```python
from build123d import *

# Parameters (mm, degrees)
F1_DEPTH  = 30.48
F2_DEPTH  = 30.48
F3_DEPTH  = 30.48
F5_DEPTH  = 661.416
F6_W      = 45.72
F6_H      = 152.3821130395
F7_DEPTH  = 222.504
F9_DEPTH  = 46.3296
F10_DEPTH = 18.288
F13_DEPTH = 296.2656
F14_DEPTH = 86.2584
F15_DEPTH = 18.288


with BuildPart() as f1:
    # F0 (on Front) → F1 (new body)
    with BuildSketch(Plane.XZ):
        Polygon((16.8911121702, 157.9167651749), (-44.0688878298, 96.9567651749), (16.8911121702, 96.9567651749), align=None)
        Polygon((16.8911121702, 96.9567651749), (-44.0688878298, 96.9567651749), (-44.0688878298, -665.0432348251), (16.8911121702, -665.0432348251), (16.8911121702, -726.0032348251), (86.011223495, -683.3165884018), (86.011223495, -646.4774608612), (43.015755713, -506.0282349586), (43.015755713, -86.7099538445), (68.1852996349, 21.7126905918), (61.4088848233, 96.9567651749), (16.8911121702, 157.9167651749), align=None)
        Polygon((16.8911121702, -665.0432348251), (-44.0688878298, -665.0432348251), (16.8911121702, -726.0032348251), align=None)
    extrude(amount=F1_DEPTH)

    # F2 (add): a face of the model
    f2_faces = [f1.faces().sort_by_distance(p)[0] for p in [
        (6.2050010019, -30.48, -294.9143233184),
    ]]
    extrude(f2_faces, amount=F2_DEPTH)

    # F3 (add): a face of the model
    f3_faces = [f1.faces().sort_by_distance(p)[0] for p in [
        (6.2050010019, -60.96, -294.9143233184),
    ]]
    extrude(f3_faces, amount=F3_DEPTH)

    # F4 (on face) → F5 (cut)
    with BuildSketch(Plane(origin=(0, 0, 0), x_dir=(-1, 0, 0), z_dir=(0, 1, 0))):
        with BuildLine():
            Line((44.0688878298, -581.2422633171), (44.0688878298, -34.1473101496))
            ThreePointArc((44.0688878298, -34.1473101496), (7.0024431669, -307.6947867334), (44.0688878298, -581.2422633171))
        make_face()
    extrude(amount=-F5_DEPTH, mode=Mode.SUBTRACT)

    # F6 (on face) → F7 (cut)
    with BuildSketch(Plane.YZ.offset(43.015755713)):
        with Locations((-68.58, -198.6809484661)):
            Rectangle(F6_W, F6_H)
    extrude(amount=-F7_DEPTH, mode=Mode.SUBTRACT)

    # F8 (on face) → F9 (cut)
    with BuildSketch(Plane(origin=(0, 0, 0), x_dir=(-1, 0, 0), z_dir=(0, 1, 0))):
        with BuildLine():
            Line((-68.1852996349, 21.7126905918), (-43.015755713, -86.7099538445))
            Line((-43.015755713, -86.7099538445), (31.0375482418, -86.7099538445))
            ThreePointArc((31.0375482418, -86.7099538445), (37.2070107283, -60.3428002224), (44.0688878298, -34.1473101496))
            Line((44.0688878298, -34.1473101496), (44.0688878298, 96.9567651749))
            Line((44.0688878298, 96.9567651749), (-16.8911121702, 157.9167651749))
            Line((-16.8911121702, 157.9167651749), (-61.4088848233, 96.9567651749))
            Line((-61.4088848233, 96.9567651749), (-68.1852996349, 21.7126905918))
        make_face()
    extrude(amount=-F9_DEPTH, mode=Mode.SUBTRACT)

    # F10 (cut): a face of the model
    f10_faces = [f1.faces().sort_by_distance(p)[0] for p in [
        (15.3196752296, 0, -444.822898096),
    ]]
    extrude(f10_faces, amount=-F10_DEPTH, mode=Mode.SUBTRACT)

    # F12 (on face) → F13 (cut)
    with BuildSketch(Plane.XZ.offset(91.44)):
        with BuildLine():
            Line((43.015755713, -390.4501199722), (43.015755713, -293.7003970146))
            ThreePointArc((43.015755713, -293.7003970146), (27.028136051, -299.6814009845), (26.5955161303, -316.7456686497))
            ThreePointArc((26.5955161303, -316.7456686497), (35.3432447647, -353.478123173), (43.015755713, -390.4501199722))
        make_face()
    extrude(amount=-F13_DEPTH, mode=Mode.SUBTRACT)

    # F11 (on face) → F14 (cut)
    with BuildSketch(Plane.YZ.offset(43.015755713)):
        with BuildLine():
            Line((-71.4861452579, -398.3681499958), (-71.4861452579, -306.9769144058))
            ThreePointArc((-71.4861452579, -306.9769144058), (-76.814746868, -292.4826164705), (-91.44, -287.5247299671))
            Line((-91.44, -287.5247299671), (-91.44, -506.0282349586))
            Line((-91.44, -506.0282349586), (-71.4861452579, -506.0282349586))
            Line((-71.4861452579, -506.0282349586), (-71.4861452579, -398.3681499958))
        make_face()
        with BuildLine():
            ThreePointArc((-27.6783167816, -287.4728058939), (-23.0664051614, -286.1317966662), (-18.288, -285.6471538544))
            Line((-18.288, -285.6471538544), (-18.288, -270.6759691181))
            ThreePointArc((-18.288, -270.6759691181), (-22.0060984175, -279.6206155123), (-27.6783167816, -287.4728058939))
        make_face()
        with BuildLine():
            Line((-44.4478472258, -398.3681499958), (-44.4478472258, -506.0282349586))
            Line((-44.4478472258, -506.0282349586), (-18.288, -506.0282349586))
            Line((-18.288, -506.0282349586), (-18.288, -285.6471538544))
            ThreePointArc((-18.288, -285.6471538544), (-23.0664051614, -286.1317966662), (-27.6783167816, -287.4728058939))
            ThreePointArc((-27.6783167816, -287.4728058939), (-33.0895793591, -292.4309253132), (-39.2827639268, -296.3690944016))
            ThreePointArc((-39.2827639268, -296.3690944016), (-42.9947480165, -303.4018680478), (-44.4478472258, -311.2202587856))
            Line((-44.4478472258, -311.2202587856), (-44.4478472258, -312.9553496838))
            Line((-44.4478472258, -312.9553496838), (-44.4478472258, -398.3681499958))
        make_face()
        with BuildLine():
            ThreePointArc((-39.2827639268, -296.3690944016), (-33.0895793591, -292.4309253132), (-27.6783167816, -287.4728058939))
            ThreePointArc((-27.6783167816, -287.4728058939), (-34.1077092685, -291.1028619629), (-39.2827639268, -296.3690944016))
        make_face()
    extrude(amount=-F14_DEPTH, mode=Mode.SUBTRACT)

    # F15 (cut): a face of the model
    f15_faces = [f1.faces().sort_by_distance(p)[0] for p in [
        (9.0527657061, -91.44, 12.1173213598),
    ]]
    extrude(f15_faces, amount=-F15_DEPTH, mode=Mode.SUBTRACT)


solid = f1.part
```
The model under review builds one solid part; all positions refer to its coordinate system, in mm. A direction names the side the tool comes from. Round coordinates to 2 decimals unless told otherwise and drop trailing zeros. Loops run counter-clockwise (first coordinate to the right, second up) from the corner with the lowest first, then second, coordinate; pieces in that order, holes last. Notation, with made-up numbers: (-12, 1) -> (39, 1) arc R12 cw to (39, 5) -> close; hole circle Ø6 at (59, -10). An arc over 180 degrees is marked (long way). Answer as a JSON object with one key per item and string values. Group by question number.
1) We need section B-B on x = 4. Write out the cut boundary in (y, z), then the cut area to 3 significant figures.
2) We need section A-A on y = -59. Write out the cut boundary in (x, z), then the cut area to 3 significant figures.
3) Mouldability with a two-part tool opening along Z and no side actions: class faces 6 (the face through (14, -18.288, -177)), 7 (the face through (39.46, -59.55, 127.01)), 8 (the face through (64.814, -54.352, -577.236)) as released by +Z, released by -Z, zero draft, split by the parting line, or undercut.
4) We need section C-C on z = -164. Write out the cut boundary in (x, y).
5) For line 1 (Y direction, x = 8, z = -29); line 2 (Z direction, x = 41.5, y = -83); line 3 (Y direction, x = 30, z = -503.5), list the stretches that pass through material, from the lowest coordinate up. Write a range as [from, to].
6) We need section D-D on z = 79. Write out the cut boundary in (x, y), then the cut area to 3 significant figures.
7) For pin 1 Ø3 at (x, y) = (-16, -45) entering from -Z; pin 2 Ø21 at (x, z) = (22.5, -374) entering from +Y; pin 3 Ø13.5 at (y, z) = (-64.5, -429.5) entering from +X, all flat-tipped, find the tip position at first contact; note any pin that passes through.
8) For faces 1 (the face through (11, -73.152, 20)), 2 (the face through (17, -71.486, -408)), 3 (the face through (18.258, -76.656, -292.64)), 4 (the face through (55.424, -59.553, -33.258)), 5 (the face through (9, -32, -506.028)), list the 3-axis set-ups (+Z, -Z, +X, -X, +Y, -Y) from which the entire face can be reached by the end or side of a thin tool; tool diameter is ignored.
Result set:
{
 "1": {"outline": "(-91.44, -713.11) -> (-18.29, -713.11) -> (-18.29, -506.03) -> (-44.45, -506.03) -> (-44.45, -311.22) arc R26.44 cw to (-27.68, -287.47) arc R41.91 ccw to (-18.29, -270.68) -> (-18.29, -86.71) -> (-46.33, -86.71) -> (-46.33, 145.03) -> (-73.15, 145.03) -> (-73.15, -122.49) -> (-45.72, -122.49) -> (-45.72, -274.87) -> (-91.44, -274.87) -> (-91.44, -287.52) arc R17.91 cw to (-71.49, -306.98) -> (-71.49, -506.03) -> (-91.44, -506.03) -> close", "area": "34,500 mm²"},
 "2": {"outline": "(-44.07, -665.04) -> (16.89, -726) -> (86.01, -683.32) -> (86.01, -646.48) -> (43.02, -506.03) -> (43.02, -390.45) arc R1294.32 ccw to (26.6, -316.75) arc R15.26 cw to (43.02, -293.7) -> (43.02, -274.87) -> (-7.53, -274.87) arc R1027.91 cw to (-44.07, -581.24) -> close; (-44.07, -34.15) arc R1027.91 cw to (-23.82, -122.49) -> (43.02, -122.49) -> (43.02, -86.71) -> (68.19, 21.71) -> (61.41, 96.96) -> (16.89, 157.92) -> (-44.07, 96.96) -> close", "area": "57,800 mm²"},
 "3": {"face 6": "zero draft", "face 7": "released by +Z", "face 8": "undercut"},
 "4": {"outline": "(-17.1, -45.72) -> (43.02, -45.72) -> (43.02, -18.29) -> (-17.1, -18.29) -> close"},
 "5": {"line 1": "[-73.15, -46.33]", "line 2": "[-710.81, -506.03], [-288.55, -274.87]", "line 3": "[-71.49, -44.45]"},
 "6": {"outline": "(-44.07, -73.15) -> (63.03, -73.15) -> (63.03, -46.33) -> (-44.07, -46.33) -> close", "area": "2,870 mm²"},
 "7": {"pin 1": "z = -694.61", "pin 2": "y = -44.45", "pin 3": "x = 43.02"},
 "8": {"face 1": "+Z, +X, -X, -Y", "face 2": "+X, -X, -Y", "face 3": "+X, -X", "face 4": "+X, +Y, -Y", "face 5": "+X, -X, +Y"}
}
